```python
from build123d import *

# Parameters (mm, degrees)
SKETCH1_W           = 58.7375
SKETCH1_H           = 19.05
BOSS_EXTRUDE1_DEPTH = 279.4
SKETCH2_W           = 88.9
SKETCH2_H           = 20.6375
CUT_EXTRUDE1_DEPTH  = 282.584420692


with BuildPart() as part:
    # Sketch1 → Boss-Extrude1 (new, symmetric)
    with BuildSketch(Plane(origin=(0, 0, 0), x_dir=(0, 0, -1), z_dir=(1, 0, 0))):
        Rectangle(SKETCH1_W, SKETCH1_H)
    extrude(amount=BOSS_EXTRUDE1_DEPTH, both=True)

    # Sketch2 → Cut-Extrude1 (cut, through all)
    with BuildSketch(Plane(origin=(0, 9.525, 0), x_dir=(1, 0, 0), z_dir=(0, 1, 0))):
        with Locations((-215.9, 0)):
            Rectangle(SKETCH2_W, SKETCH2_H)
        with Locations((215.9, 0)):
            Rectangle(SKETCH2_W, SKETCH2_H)
        with Locations((-107.95, 0)):
            Rectangle(SKETCH2_W, SKETCH2_H)
        Rectangle(SKETCH2_W, SKETCH2_H)
        with Locations((107.95, 0)):
            Rectangle(SKETCH2_W, SKETCH2_H)
    extrude(amount=-CUT_EXTRUDE1_DEPTH, mode=Mode.SUBTRACT)


solid = part.part
```
Design review of the part built by this model. Coordinates are the model's own, in mm. A direction names the side the tool comes from. Coordinates: 2 decimals unless noted, no trailing zeros. Order: outer loops, then holes, each group sorted by start corner. A loop starts at its lowest first (then second) coordinate and runs counter-clockwise, first axis right, second up.
1) Wall thickness on line 1 along X through (y, z) = (-4, 9); line 2 along Z through (x, y) = (21.5, 1): over which ranges is each line inside the solid? List them lowest first.
2) Take a section at B-B, the plane x = 128. Give the boundary of the cut face in (y, z) (3 decimals).
3) For faces 4 (the flat face through (-279.4, 0, 0)), 5 (the flat face through (215, 0, 10.319)), list the 3-axis set-ups (+Z, -Z, +X, -X, +Y, -Y) from which the entire face can be reached by the end or side of a thin tool; tool diameter is ignored.
4) Mouldability with a two-part tool opening along Z and no side actions: class faces 1 (the flat face through (4, 0, -29.369)), 2 (the flat face through (-217, 0, -10.319)), 3 (the flat face through (279.4, 0, 0)) as +Z half, -Z half, draft (parallel to the pull), parting line (faces both ways), or undercut.
5) Take a section at A-A, the plane y = 1. Give the boundary of the cut face in (x, z), and give its area (3 significant figures).
Returned:
1. line 1: x = -279.4 to -260.35, -171.45 to -152.4, -63.5 to -44.45, 44.45 to 63.5, 152.4 to 171.45, 260.35 to 279.4
1. line 2: z = -29.37 to -10.32, 10.32 to 29.37
2. outline: (-9.525, -29.369) - (9.525, -29.369) - (9.525, -10.319) - (-9.525, -10.319) - close; (-9.525, 10.319) - (9.525, 10.319) - (9.525, 29.369) - (-9.525, 29.369) - close
3. face 4: +Z, -Z, -X, +Y, -Y
3. face 5: +Y, -Y
4. face 1: -Z half
4. face 2: undercut
4. face 3: draft
5. outline: (-279.4, -29.37) - (279.4, -29.37) - (279.4, 29.37) - (-279.4, 29.37) - close; hole (-260.35, -10.32) - (-171.45, -10.32) - (-171.45, 10.32) - (-260.35, 10.32) - close; hole (-152.4, -10.32) - (-63.5, -10.32) - (-63.5, 10.32) - (-152.4, 10.32) - close; hole (-44.45, -10.32) - (44.45, -10.32) - (44.45, 10.32) - (-44.45, 10.32) - close; hole (63.5, -10.32) - (152.4, -10.32) - (152.4, 10.32) - (63.5, 10.32) - close; hole (171.45, -10.32) - (260.35, -10.32) - (260.35, 10.32) - (171.45, 10.32) - close
5. area: 23,600 mm2
